Check sheet for the drawn part. Datum: minimum x, y, z corner. Units: mm. Round coordinates to 2 decimals unless told otherwise and drop trailing zeros. Write each loop counter-clockwise with the first axis right and the second up, starting at its lowest first coordinate (ties: lowest second). Pieces come first, ordered by that corner, then holes. Notation, with made-up numbers: M -13.75,62.5 L 40.25,62.5 A32 ccw 40.25,91.5 Z; hole C -8.5,-17.75 d1. An arc over 180 degrees is marked long. Put each result on its own line as item: value.
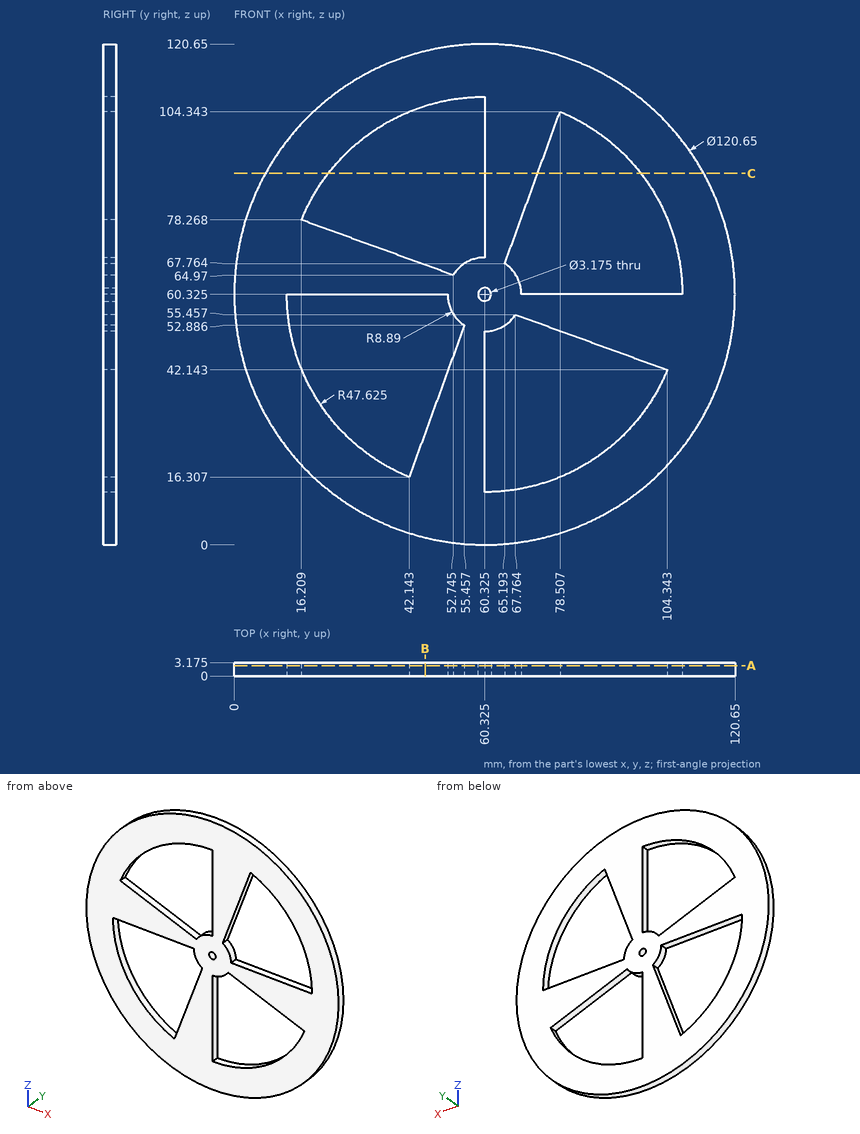
1. Depth check by flat-ended pin: pin 1 Ø1.6 at (x, y) = (85.5, 2) entering from +Z; pin 2 Ø1 at (x, y) = (41, 2.5) entering from -Z; pin 3 Ø1.5 at (y, z) = (2.5, 49) entering from -X. Enter the tip coordinate at first touch or a pass-through.
Computed values:
pin 1: stops at z = 115.51
pin 2: stops at z = 3.01
pin 3: stops at x = 0.93
2. Scan lines: probe 1 along X at (y, z) = (1.6, 21.5) (1 decimal); probe 2 along Z at (x, y) = (26, 2.1) (1 decimal); probe 3 along Z at (x, y) = (85.5, 0.9) (1 decimal). Record each from-to range of solid material in increasing order.
Computed values:
probe 1: x = 14.2 to 32.7, 44 to 60.3, 87.9 to 106.5
probe 2: z = 10.7 to 27.3, 60.3 to 74.7, 93.3 to 109.9
probe 3: z = 5.5 to 19.9, 49 to 60.3, 100.8 to 115.1
3. Cross-section at B-B (x = 46). Enter the section's corners in (y, z) (1 decimal), then the cut area to 3 significant figures.
Computed values:
outline: M 0,1.7 L 3.2,1.7 L 3.2,26.9 L 0,26.9 Z; M 0,60.3 L 3.2,60.3 L 3.2,67.4 L 0,67.4 Z; M 0,105.7 L 3.2,105.7 L 3.2,118.9 L 0,118.9 Z
area: 144 mm2
4. Cross-section at A-A (y = 2.5). Count the separate pieces of the cut face and the enclosed holes in it, then the cut area to 3 significant figures.
Computed values:
separate pieces: 1
enclosed holes: 5
area: 6,380 mm2
5. Cross-section at C-C (z = 89.5). Enter the section's corners in (x, y) (1 decimal), then the cut area to 3 significant figures.
Computed values:
outline: M 7.5,0 L 22.7,0 L 22.7,3.2 L 7.5,3.2 Z; M 60.3,0 L 73.1,0 L 73.1,3.2 L 60.3,3.2 Z; M 98,0 L 113.1,0 L 113.1,3.2 L 98,3.2 Z
area: 137 mm2
